Autodesk Inventor part; units mm, degrees
ref_plane "YZ Plane" through (0, 0, 0) normal (1, 0, 0) x (0, 1, 0)
ref_plane "XZ Plane" through (0, 0, 0) normal (0, 1, 0) x (-1, 0, 0)
ref_plane "XY Plane" through (0, 0, 0) normal (0, 0, 1) x (1, 0, 0)
sketch "Profile" plane through (0, 0, 0) normal (0, 0, 1) x (1, 0, 0)
  line L0 (-8.4, 0) -> (-8.4, 11)
  line L1 (-8.4, 11) -> (0, 11)
  line L2 (0, 11) -> (0.5774, 12)
  line L3 (0.5774, 12) -> (18.0774, 12)
  line L4 (18.0774, 12) -> (18.6547, 11)
  line L5 (18.6547, 11) -> (26.6, 11)
  line L6 (26.6, 11) -> (26.6, 0)
  line L7 (-8.4, 0) -> (0, 0)
  line L8 (0, 0) -> (0, 9)
  line L9 (0, 9) -> (18.6, 9)
  line L10 (18.6, 9) -> (18.6, 0)
  line L11 (18.6, 0) -> (26.6, 0)
  line L12 (-15.4, 0) -> (33.6, 0) construction
  line L13 (0, 11) -> (0, 9) construction
  dimension "BodyLength" = 35
  dimension "d1" = 11
  dimension "d3" = 120
  dimension "d4" = 120
  dimension "d5" = 17.5
  dimension "d6" = 8.4
  dimension "d16" = 8
  dimension "d29" = 1
  dimension "d30" = 9
revolve "ProfileRevolveFeature" add sketch "Profile" angle 360 about axis through (-10, 0, 0) along (1, 0, 0)
sketch "InsideHole" plane through (-8.4, 0, 0) normal (-1, 0, 0) x (0, 0, 1)
  circle A0 centre (0, 0) radius 9 construction
hole "InsideHoleFeature" at (-8.4, 0, 0) direction (1, 0, 0) diameter 19 end through all
chamfer "EndChamferFeature" distance 1 angle 45 1 edges at (-8.4, -11, 0)
sketch "CapMountHole" plane through (0, 0, 0) normal (0, 1, 0) x (-1, 0, 0)
  line L0 (-26.6, 11) -> (-26.6, -11) construction
  line L1 (7.6, 0) -> (-45.6, 0) construction
  circle A0 centre (-22.1, 0) radius 1.25
  point P0 (0, 0)
  dimension "d31" = 4.5
  dimension "d39" = 2.5
extrude "CapMountHoleFeature" cut sketch "CapMountHole" along normal through all both and the other way through all
equation "\"d5\" = 0.5 * BodyLength"
equation "\"d6\" = 0.24 * BodyLength"
properties part number "BackPair1PistonBody"
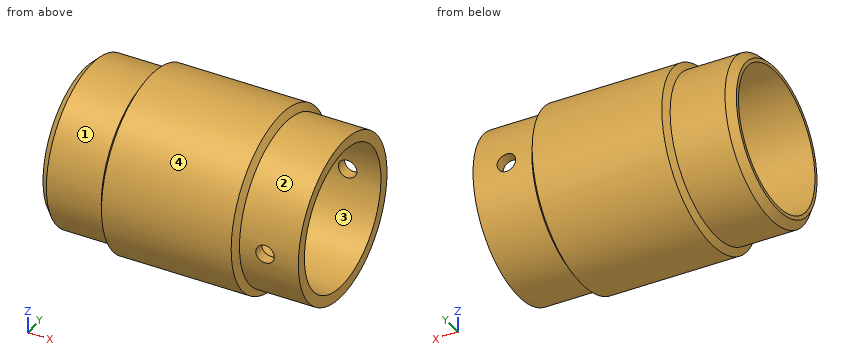
Can you work these out from the model? Positions are in its coordinate system, mm. Face numbers are marked on the shaded views. A direction names the side the tool comes from. Round coordinates to 2 decimals unless told otherwise and drop trailing zeros. Loops run counter-clockwise (first coordinate to the right, second up) from the corner with the lowest first, then second, coordinate; pieces in that order, holes last. Notation, with made-up numbers: (44.5, 2) - (94.5, 2) arc R23 cw to (94.5, 33) - close; hole circle Ø5 at (52.5, 41). An arc over 180 degrees is marked (long way). Answer in a Markdown table with one row per item. Add a question column.
Q1. We'd pull the mould along Y, two halves only. Please class the marked faces 3 and 4: pulls with the +Y half, pulls with the -Y half, needs draft (parallel to the pull), parting line crosses it, or undercut.
Q2. I want a section at A-A on z = 0. List the corners of the cut face in (x, y) for me.
Q3. I want a section at B-B on x = 22.1. List the corners of the cut face in (y, z) for me, and give its area (3 significant figures).
Q4. I want a section at D-D on x = 3. List the corners of the cut face in (y, z) for me, and give its area (3 significant figures).
Q5. For pin 1 Ø1 at (x, y) = (16.5, -9.5) entering from -Z; pin 2 Ø1 at (x, y) = (10.5, -5) entering from +Z; pin 3 Ø6 at (x, y) = (21, 6) entering from -Z, each with a flat end and sliding along its axis, tell me the tip position at first contact or that it passes through.
Q6. I need wall thicknesses on L1, parallel to Z at x = 15, y = -0.25; L2, parallel to X at y = 10, z = 0. Which ranges of each line are inside material? Lowest first, please.
Q7. Which directions (+Z, -Z, +X, -X, +Y, -Y) give clear straight access to the entire face, cutting with the end or side of a thin tool? Please do the marked faces 1 and 2.
Q8. I want a section at C-C on y = 0. List the corners of the cut face in (x, z) for me, and give its area (3 significant figures).
A:
| question | item | result |
|---|---|---|
| 1 | face 3 | undercut |
| 1 | face 4 | parting line crosses it |
| 2 | outline | (-8.4, -10) - (-7.4, -11) - (0, -11) - (0.58, -12) - (18.08, -12) - (18.65, -11) - (20.85, -11) - (20.85, -9.5) - (-8.4, -9.5) - close; (-8.4, 9.5) - (20.85, 9.5) - (20.85, 11) - (18.65, 11) - (18.08, 12) - (0.58, 12) - (0, 11) - (-7.4, 11) - (-8.4, 10) - close; (23.35, -11) - (26.6, -11) - (26.6, -9.5) - (23.35, -9.5) - close; (23.35, 9.5) - (26.6, 9.5) - (26.6, 11) - (23.35, 11) - close |
| 3 | outline | (-10.93, -1.25) arc R11 ccw to (10.93, -1.25) - (9.42, -1.25) arc R9.5 cw to (-9.42, -1.25) - close; (-10.93, 1.25) - (-9.42, 1.25) arc R9.5 cw to (9.42, 1.25) - (10.93, 1.25) arc R11 ccw to start |
| 3 | area | 89.1 mm^2 |
| 4 | outline | circle Ø24 at (0, 0); hole circle Ø19 at (0, 0) |
| 4 | area | 169 mm^2 |
| 5 | pin 1 | z = -7.94 |
| 5 | pin 2 | z = 11.12 |
| 5 | pin 3 | z = -10.76 |
| 6 | L1 | -12 to -9.5, 9.5 to 12 |
| 6 | L2 | -8.4 to 20.85, 23.35 to 26.6 |
| 7 | face 1 | -X |
| 7 | face 2 | +X |
| 8 | outline | (-8.4, -10) - (-7.4, -11) - (0, -11) - (0.58, -12) - (18.08, -12) - (18.65, -11) - (26.6, -11) - (26.6, -9.5) - (-8.4, -9.5) - close; (-8.4, 9.5) - (26.6, 9.5) - (26.6, 11) - (18.65, 11) - (18.08, 12) - (0.58, 12) - (0, 11) - (-7.4, 11) - (-8.4, 10) - close |
| 8 | area | 140 mm^2 |
